Design review of the part built by this model. Coordinates are the model's own, in mm. A direction names the side the tool comes from. Give positions to 0.01 mm unless a question says otherwise; leave off trailing zeros. Write each loop counter-clockwise with the first axis right and the second up, starting at its lowest first coordinate (ties: lowest second). Pieces come first, ordered by that corner, then holes. Notation, with made-up numbers: (27, 71.5) -> (37, 71.5) arc R20 ccw to (37, 87.5) -> close; hole circle Ø8 at (12.25, 50.5). An arc over 180 degrees is marked (long way). Write each question's results on one line, items separated by ' | '. Start each with the question number.
(1) Take a section at B-B (z = 0). State the section outline as (x, y) points, plus the area to 3 significant figures.
(2) Take a section at A-A (y = 2.5). State the section outline as (x, z) points.
(3) To check wall thickness, follow probe 1 along Z at (x, y) = (-3.75, 4.8); probe 2 along Z at (x, y) = (0, 1.25); probe 3 along X at (y, z) = (2.45, 52). State the ranges of each line that lie inside material, in increasing order.
(4) Take a section at D-D (z = 35). State the section outline as (x, y) points.
(5) Take a section at C-C (x = -3). State the section outline as (y, z) points.
(6) For faces 4 (the face through (-2, 2, -3)), 5 (the face through (-2, 2, 3)), 6 (the face through (3, 3, 5.656)), list the 3-axis set-ups (+Z, -Z, +X, -X, +Y, -Y) from which the entire face can be reached by the end or side of a thin tool; tool diameter is ignored.
(7) Clearance check with flat-ended pins moving along their axes: pin 1 (1.5 mm diameter, centred on x = 2, z = 44.5, fed in from +Y); pin 2 (3 mm diameter, centred on x = 4.5, y = 2.5, fed in from -Z). State where each tip first meets the part, or that it passes through.
(8) Mouldability with a two-part tool opening along X and no side actions: class faces 1 (the face through (-1.95, 2.46, -0.26)), 2 (the face through (-6.93, 2.46, 0.07)), 3 (the face through (6, 2, 79.656)) as released by +X, released by -X, zero draft, split by the parting line, or undercut.
from build123d import *

# Parameters (mm, degrees)
SKETCH_2_R          = 2
EXTRUDE_2_DEPTH     = 5
EXTRUDE_3_DEPTH     = 5
SKETCH_4_OUTSIDE_W  = 34.301
SKETCH_4_OUTSIDE_H  = 23.848
SKETCH_4_OUTSIDE_R  = 2
CUT_EXTRUDE_1_DEPTH = 74


with BuildPart() as part:
    # 草图2 → 凸台-拉伸2 (new body)
    with BuildSketch(Plane(origin=(0, 0, 0), x_dir=(1, 0, 0), z_dir=(0, 1, 0))):
        with BuildLine():
            Line((-3.932336285, 3), (0.337762879, 3))
            Line((0.337762879, 3), (0.337762879, -3))
            Line((0.337762879, -3), (-3.932336285, -3))
            ThreePointArc((-3.932336285, -3), (-6.932336285, 0), (-3.932336285, 3))
        make_face()
        with Locations(Location((-3.932336285, 0, 0), (0, 0, 270))):
            Circle(SKETCH_2_R, mode=Mode.SUBTRACT)
    extrude(amount=EXTRUDE_2_DEPTH)

    # 草图3 → 凸台-拉伸3 (add)
    with BuildSketch(Plane(origin=(0, 0, 0), x_dir=(1, 0, 0), z_dir=(0, 1, 0))):
        with BuildLine():
            Line((2.537654461, -79.655778605), (8.520746385, -79.655778605))
            Line((8.520746385, -79.655778605), (8.520746385, -8.429696767))
            Line((8.520746385, -8.429696767), (8.520746385, -5.525308021))
            ThreePointArc((8.520746385, -5.525308021), (6.143965834, 0.383204819), (0.337762879, 3))
            Line((0.337762879, 3), (0.337762879, -3))
            ThreePointArc((0.337762879, -3), (1.910553846, -3.850740646), (2.537654461, -5.525308021))
            Line((2.537654461, -5.525308021), (2.537654461, -8.429696767))
            Line((2.537654461, -8.429696767), (2.537654461, -79.655778605))
        make_face()
    extrude(amount=EXTRUDE_3_DEPTH)

    # 草图4 outside → 切除-拉伸1 (cut)
    with BuildSketch(Plane.XY.offset(79.655778605)):
        with Locations((0.7945, 2.5)):
            Rectangle(SKETCH_4_OUTSIDE_W, SKETCH_4_OUTSIDE_H)
        with Locations((5.529200423, 2.5)):
            Circle(SKETCH_4_OUTSIDE_R, mode=Mode.SUBTRACT)
    extrude(amount=-CUT_EXTRUDE_1_DEPTH, mode=Mode.SUBTRACT)


solid = part.part
Report:
1) outline: (-6.93, 0) -> (-5.93, 0) -> (-5.93, 5) -> (-6.93, 5) -> close; (-1.93, 0) -> (6.49, 0) -> (6.49, 5) -> (-1.93, 5) -> close | area: 47.1 mm2
2) outline: (-3.93, -3) -> (0.34, -3) arc R8.53 ccw to (8.52, 5.53) -> (8.52, 5.66) -> (7.53, 5.66) -> (7.53, 79.66) -> (3.53, 79.66) -> (3.53, 5.66) -> (2.54, 5.66) -> (2.54, 5.53) arc R2.55 cw to (0.34, 3) -> (-3.93, 3) arc R3 ccw to start; hole circle Ø4 at (-3.93, 0)
3) probe 1: -3 to -1.99, 1.99 to 3 | probe 2: -3 to 3 | probe 3: 3.53 to 7.53
4) outline: circle Ø4 at (5.53, 2.5)
5) outline: (0, -3) -> (5, -3) -> (5, -1.77) -> (0, -1.77) -> close; (0, 1.77) -> (5, 1.77) -> (5, 3) -> (0, 3) -> close
6) face 4: -Z, +X, -X, +Y, -Y | face 5: +Z, -X, +Y, -Y | face 6: +Z
7) pin 1: through | pin 2: z = -2.46
8) face 1: undercut | face 2: released by -X | face 3: zero draft
